Design review of the part built by this model. Coordinates are the model's own, in mm. A direction names the side the tool comes from. Give positions to 0.01 mm unless a question says otherwise; leave off trailing zeros. Write each loop counter-clockwise with the first axis right and the second up, starting at its lowest first coordinate (ties: lowest second). Pieces come first, ordered by that corner, then holes.
```python
from build123d import *

# Parameters (mm, degrees)
SKETCH1_W             = 110
SKETCH1_H             = 80
BOSS_EXTRUDE1_DEPTH   = 12.5
SKETCH2_W             = 110
SKETCH2_H             = 30
BOSS_EXTRUDE2_DEPTH   = 60
SKETCH3_W             = 40
SKETCH3_H             = 25
CUT_EXTRUDE1_DEPTH    = 104.832798286
CHAMFER1_SIZE         = 3
FILLET1_R             = 6
F_1_0MM_DOWEL_HOLE1_D = 15


with BuildPart() as part:
    # Sketch1 → Boss-Extrude1 (new, symmetric)
    with BuildSketch(Plane(origin=(0, 0, 0), x_dir=(1, 0, 0), z_dir=(0, 1, 0))):
        Rectangle(SKETCH1_W, SKETCH1_H)
    extrude(amount=BOSS_EXTRUDE1_DEPTH, both=True)

    # Sketch2 → Boss-Extrude2 (add)
    with BuildSketch(Plane(origin=(0, 12.5, 0), x_dir=(1, 0, 0), z_dir=(0, 1, 0))):
        with Locations((0, -25)):
            Rectangle(SKETCH2_W, SKETCH2_H)
    extrude(amount=BOSS_EXTRUDE2_DEPTH)

    # Sketch3 → Cut-Extrude1 (cut, through all)
    with BuildSketch(Plane(origin=(0, 0, 10), x_dir=(-1, 0, 0), z_dir=(0, 0, -1))):
        with Locations((0, 60)):
            Rectangle(SKETCH3_W, SKETCH3_H)
    extrude(amount=-CUT_EXTRUDE1_DEPTH, mode=Mode.SUBTRACT)

    # Chamfer1
    chamfer1_edges = [part.edges().sort_by_distance(p)[0] for p in [
        (-55, 72.5, 25),
        (55, 72.5, 25),
        (20, 72.5, 25),
        (-20, 72.5, 25),
    ]]
    chamfer(chamfer1_edges, length=CHAMFER1_SIZE)

    # Fillet1
    fillet1_edges = [part.edges().sort_by_distance(p)[0] for p in [
        (-55, 0, -40),
        (55, 0, -40),
    ]]
    fillet(fillet1_edges, radius=FILLET1_R)

    # Ø1.0mm Dowel Hole1 (through all)
    with Locations(Plane(origin=(0, 12.5, 0), x_dir=(1, 0, 0), z_dir=(0, 1, 0))):
        with Locations((25, 15), (-25, 15)):
            Hole(F_1_0MM_DOWEL_HOLE1_D / 2)


solid = part.part
```
(1) Consider section B-B, the plane y = 7. Give the boundary of the cut face in (x, z).
Resolved:
outline: (-55, -34) arc R6 ccw to (-49, -40) - (49, -40) arc R6 ccw to (55, -34) - (55, 40) - (-55, 40) - close; hole circle Ø15 at (-25, -15); hole circle Ø15 at (25, -15)
(2) Clearance check with flat-ended pins moving along their axes: P1, Ø12, axis at x = 25, z = -15, coming from the -Y side; P2, Ø19.5, axis at x = -25, z = -15, coming from the +Y side. State where each tip first meets the part, or that it passes through.
Resolved:
P1: passes through
P2: stops at y = 12.5
(3) Consider section D-D, the plane y = 55.5. Give the boundary of the cut face in (x, z).
Resolved:
outline: (-55, 10) - (-20, 10) - (-20, 40) - (-55, 40) - close; (20, 10) - (55, 10) - (55, 40) - (20, 40) - close
(4) To check wall thickness, follow L1, parallel to Z at x = 25, y = -5; L2, parallel to Z at x = 3.5, y = 17.5; L3, parallel to Y at x = 29.5, z = -31. State the ranges of each line that lie inside material, in increasing order.
Resolved:
L1: z = -40 to -22.5, -7.5 to 40
L2: z = 10 to 40
L3: y = -12.5 to 12.5
(5) Mouldability with a two-part tool opening along Z and no side actions: class faces 4 (the face through (32.493, -0.175, -15.33)), 5 (the face through (-1, 0, -40)), 6 (the face through (-20, 58, 25)) as pulls with the +Z half, pulls with the -Z half, needs draft (parallel to the pull), parting line crosses it, or undercut.
Resolved:
face 4: undercut
face 5: pulls with the -Z half
face 6: needs draft
(6) Consider section C-C, the plane x = 25. Give the boundary of the cut face in (y, z).
Resolved:
outline: (-12.5, -40) - (12.5, -40) - (12.5, -22.5) - (-12.5, -22.5) - close; (-12.5, -7.5) - (12.5, -7.5) - (12.5, 10) - (72.5, 10) - (72.5, 40) - (-12.5, 40) - close
(7) Consider section A-A, the plane z = -15. Give the boundary of the cut face in (x, y).
Resolved:
outline: (-55, -12.5) - (-32.5, -12.5) - (-32.5, 12.5) - (-55, 12.5) - close; (-17.5, -12.5) - (17.5, -12.5) - (17.5, 12.5) - (-17.5, 12.5) - close; (32.5, -12.5) - (55, -12.5) - (55, 12.5) - (32.5, 12.5) - close
(8) Tool access review of faces 1 (the face through (55, 19, 12)), 2 (the face through (21.5, 71, 24.8)), 3 (the face through (-1, 12.5, -15)): name each direction out of +Z, -Z, +X, -X, +Y, -Y from which nothing blocks a thin tool from reaching the whole face with its end or side.
Resolved:
face 1: +Z, -Z, +X, +Y, -Y
face 2: +Z, -Z, +Y
face 3: -Z, +X, -X, +Y
